Read the model definition and answer for the solid it produces. Units are mm, in the model's axes. A direction names the side the tool comes from. Give positions to 0.01 mm unless a question says otherwise; leave off trailing zeros. Loops run counter-clockwise (first coordinate to the right, second up) from the corner with the lowest first, then second, coordinate; pieces in that order, holes last. Notation, with made-up numbers: (49, -1.5) - (90, -1.5) arc R14 ccw to (90, 19.5) - close; hole circle Ø10 at (-36, 7.5). An arc over 180 degrees is marked (long way). Use a Markdown table: item, result. Add a question column.
Item 1: A cutting plane is placed at A-A (y = 0). Determine the outline of the cut face in (x, z), plus the area to 3 significant figures.
Item 2: A cutting plane is placed at D-D (z = 26). Determine the outline of the cut face in (x, y), plus the area to 3 significant figures.
Item 3: A cutting plane is placed at C-C (z = 12.5). Determine the outline of the cut face in (x, y), plus the area to 3 significant figures.
Item 4: Consider probe 1 along Z at (x, y) = (-7, 7.5); probe 2 along Z at (x, y) = (1.25, -2); probe 3 along Y at (x, z) = (-9, 0). Determine where each line is inside the solid, lowest interval first. Write a range as [from, to].
Item 5: Which of the six approach directions +Z, -Z, +X, -X, +Y, -Y give full straight-line access (tool end or side, diameter ignored) to faces 1 (the face through (2, 2, 26.964)), 2 (the face through (-1.5, 0, 35)), 3 (the face through (-3.755, -11.923, -0.886))?
Item 6: Each of these flat-tipped pins is pushed along its axis until it touches: P1, Ø1.5, axis at x = -7.5, z = 0, coming from the -Y side; P2, Ø2, axis at y = 0.5, z = 35, coming from the -X side; P3, Ø8, axis at x = -9, z = 11, coming from the +Y side; P4, Ø8, axis at x = 7, z = 29.5, coming from the -Y side. Where does it stop, or does it pass through?
Item 7: A cutting plane is placed at B-B (x = 0). Determine the outline of the cut face in (y, z).
from build123d import *

# Parameters (mm, degrees)
F3_DEPTH = 8


with BuildPart() as f1:
    # F0 (on Right) → F1 (revolve)
    with BuildSketch(Plane.YZ):
        Polygon((-12.5, -25.536002), (0, -25.536002), (0, 38.963998), (-2, 38.963998), (-2, 26.963998), (-3.5, 26.963998), (-3.5, 24.463998), (-12.5, 24.463998), align=None)
    revolve(axis=Axis((0, 0, 6.713998), (0, 0, -1)))

    # F2 (on face) → F3 (cut)
    with BuildSketch(Plane.XY.offset(38.963998)):
        with BuildLine():
            Line((-1.5, -1.322876), (-1.5, 1.322876))
            ThreePointArc((-1.5, 1.322876), (-2, 0), (-1.5, -1.322876))
        make_face()
    extrude(amount=-F3_DEPTH, mode=Mode.SUBTRACT)


solid = f1.part
Geometry says:
| question | item | result |
|---|---|---|
| 1 | outline | (-12.5, -25.54) - (12.5, -25.54) - (12.5, 24.46) - (3.5, 24.46) - (3.5, 26.96) - (2, 26.96) - (2, 38.96) - (-1.5, 38.96) - (-1.5, 30.96) - (-2, 30.96) - (-2, 26.96) - (-3.5, 26.96) - (-3.5, 24.46) - (-12.5, 24.46) - close |
| 1 | area | 1,310 mm² |
| 2 | outline | circle Ø7 at (0, 0) |
| 2 | area | 38.5 mm² |
| 3 | outline | circle Ø25 at (0, 0) |
| 3 | area | 491 mm² |
| 4 | probe 1 | [-25.54, 24.46] |
| 4 | probe 2 | [-25.54, 26.96] |
| 4 | probe 3 | [-8.67, 8.67] |
| 5 | face 1 | +Z |
| 5 | face 2 | +Z, -X, +Y, -Y |
| 5 | face 3 | +Z, -Z |
| 6 | P1 | y = -10.52 |
| 6 | P2 | x = -1.5 |
| 6 | P3 | y = 11.46 |
| 6 | P4 | through |
| 7 | outline | (-12.5, -25.54) - (12.5, -25.54) - (12.5, 24.46) - (3.5, 24.46) - (3.5, 26.96) - (2, 26.96) - (2, 38.96) - (-2, 38.96) - (-2, 26.96) - (-3.5, 26.96) - (-3.5, 24.46) - (-12.5, 24.46) - close |
